```python
from build123d import *

# Parameters (mm, degrees)
SKETCH_R     = 12.715244
SKETCH_W     = 6
SKETCH_H     = 20
PAD_DEPTH    = 50
SKETCH001_R  = 5
POCKET_DEPTH = 30


with BuildPart() as part:
    # Sketch → Pad (new body)
    with BuildSketch(Plane.XY):
        with Locations((-51, 27)):
            Circle(SKETCH_R)
        with Locations((-51, 27)):
            Rectangle(SKETCH_W, SKETCH_H, mode=Mode.SUBTRACT)
    extrude(amount=PAD_DEPTH)

    # Sketch001 (on Face7 of Pad) → Pocket (cut)
    with BuildSketch(Plane.XY.offset(50)):
        with Locations((-51, 27)):
            Circle(SKETCH001_R)
    extrude(amount=-POCKET_DEPTH, mode=Mode.SUBTRACT)


solid = part.part
```
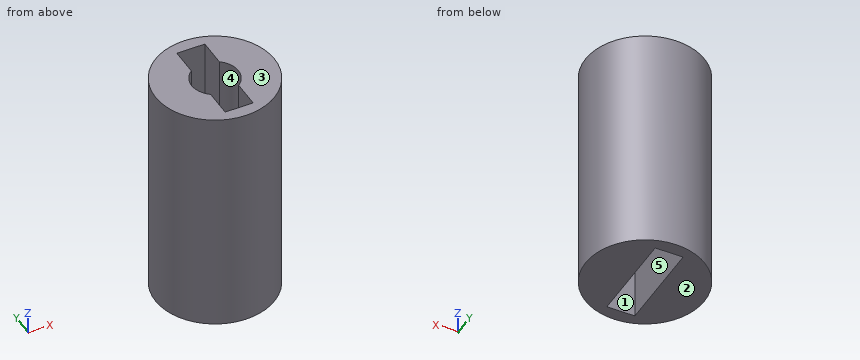
CAD build for the part. Positions are in the model's coordinates, mm. Face numbers are marked on the shaded views. A direction names the side the tool comes from. Give positions to 0.01 mm unless a question says otherwise; leave off trailing zeros. Write each loop counter-clockwise with the first axis right and the second up, starting at its lowest first coordinate (ties: lowest second). Pieces come first, ordered by that corner, then holes. Notation, with made-up numbers: M 18.25,37 L 54.25,37 A22 cw 54.25,73 Z; hole C 23,27.25 d6. An arc over 180 degrees is marked long. Return JSON: item names as keys, results as strings. Group by question number.
(1) Mould opens along Z. For the marked faces 1, 2 and 3 say: pulls with the +Z half, pulls with the -Z half, needs draft (parallel to the pull), parting line crosses it, or undercut.
(2) 3-axis set-ups, long thin cutter, end or side, ignore diameter. For the marked faces 4 and 5: which of +Z, -Z, +X, -X, +Y, -Y reach the whole face in a straight line?
(3) Drill centre lines: L1, parallel to Y at x = -48.75, z = 29.5; L2, parallel to X at y = 21.5, z = 16; L3, parallel to X at y = 19.75, z = 10.5. Where is each one in solid material? Low to high. Write a range as [from, to].
(4) Band-saw the part on B-B (x = -51). Give the cut face in (y, z), and give its area (3 significant figures).
(5) Band-saw the part on C-C (z = 40). Give the cut face in (x, y).
(6) Band-saw the part on D-D (y = 19.25). Give the cut face in (x, z), and give its area (3 significant figures).
(7) Band-saw the part on A-A (y = 27). Give the cut face in (x, z).
(8) Flat gauge pins, fed straight in: pin 1 Ø2 at (y, z) = (18, 35) entering from -X; pin 2 Ø0.6 at (x, y) = (-54.5, 29) entering from +Z; pin 3 Ø6 at (y, z) = (32, 23) entering from -X. Where does each tip first touch, or does it go through?
Entries:
{
 "1": {"face 1": "needs draft", "face 2": "pulls with the -Z half", "face 3": "pulls with the +Z half"},
 "2": {"face 4": "+Z", "face 5": "+Z, -Z"},
 "3": {"L1": "y = [14.49, 17], [37, 39.51]", "L2": "x = [-62.46, -54], [-48, -39.54]", "L3": "x = [-61.45, -54], [-48, -40.55]"},
 "4": {"outline": "M 14.28,0 L 17,0 L 17,50 L 14.28,50 Z; M 37,0 L 39.72,0 L 39.72,50 L 37,50 Z", "area": "272 mm^2"},
 "5": {"outline": "C -51,27 d25.43; hole M -54,17 L -48,17 L -48,23 A5 ccw -48,31 L -48,37 L -54,37 L -54,31 A5 ccw -54,23 Z"},
 "6": {"outline": "M -61.08,0 L -54,0 L -54,50 L -61.08,50 Z; M -48,0 L -40.92,0 L -40.92,50 L -48,50 Z", "area": "708 mm^2"},
 "7": {"outline": "M -63.72,0 L -54,0 L -54,20 L -56,20 L -56,50 L -63.72,50 Z; M -48,0 L -38.28,0 L -38.28,50 L -46,50 L -46,20 L -48,20 Z"},
 "8": {"pin 1": "stops at x = -60.88", "pin 2": "stops at z = 20", "pin 3": "stops at x = -63.56"}
}
